For this review, take the finished solid that the model builds, in its own axes (mm). A direction names the side the tool comes from. Coordinates: 2 decimals unless noted, no trailing zeros. Loops run counter-clockwise (first coordinate to the right, second up) from the corner with the lowest first, then second, coordinate; pieces in that order, holes last. Notation, with made-up numbers: (78.25, 26.25) -> (111.25, 26.25) arc R21 cw to (111.25, 62.25) -> close; hole circle Ø4 at (-25.75, -17). An arc over 180 degrees is marked (long way). Use a Markdown table: item, result.
from build123d import *

# Parameters (mm, degrees)
SKETCH1_W               = 203.2
SKETCH1_H               = 0.889
SKETCH2_W               = 101.6
SKETCH2_H               = 16.721370504
CUT_EXTRUDE1_DEPTH      = 10.525
CUT_EXTRUDE1_DEPTH_BACK = 10.525


with BuildPart() as part:
    # Sketch1 → Revolve1 (revolve)
    with BuildSketch(Plane(origin=(0, 0, 0), x_dir=(1, 0, 0), z_dir=(0, 1, 0))):
        with Locations((101.6, 9.0805)):
            Rectangle(SKETCH1_W, SKETCH1_H)
    revolve(axis=Axis((0, 0, 0), (1, 0, 0)))

    # Sketch2 → Cut-Extrude1 (cut, two sides)
    with BuildSketch(Plane.XY) as cut_extrude1_sk:
        with Locations((101.6, 8.360685252)):
            Rectangle(SKETCH2_W, SKETCH2_H)
    extrude(amount=CUT_EXTRUDE1_DEPTH, mode=Mode.SUBTRACT)
    extrude(cut_extrude1_sk.sketch, amount=-CUT_EXTRUDE1_DEPTH_BACK, mode=Mode.SUBTRACT)


solid = part.part
(1) Take a section at D-D on x = 170.5. Write out the cut boundary in (y, z) (3 decimals).
Found:
| item | result |
|---|---|
| outline | circle Ø19.05 at (0, 0); hole circle Ø17.272 at (0, 0) |
(2) For pin 1 Ø7.5 at (y, z) = (6.5, 0.5) entering from +X; pin 2 Ø3 at (x, z) = (46.5, 2) entering from +Y, all flat-tipped, find the tip position at first contact; note any pin that passes through.
Found:
| item | result |
|---|---|
| pin 1 | stops at x = 203.2 |
| pin 2 | stops at y = 9.51 |
(3) Mouldability with a two-part tool opening along X and no side actions: class faces 1 (the face through (103.02, -9.3, 2.06)), 2 (the face through (0, -8, 4)), 3 (the face through (50.8, 9, -1)) as pulls with the +X half, pulls with the -X half, needs draft (parallel to the pull), parting line crosses it, or undercut.
Found:
| item | result |
|---|---|
| face 1 | needs draft |
| face 2 | pulls with the -X half |
| face 3 | undercut |
(4) Take a section at A-A on z = 0. Write out the cut boundary in (x, y) (3 decimals), plus the area to 3 significant figures.
Found:
| item | result |
|---|---|
| outline | (0, -9.525) -> (203.2, -9.525) -> (203.2, -8.636) -> (0, -8.636) -> close; (0, 8.636) -> (50.8, 8.636) -> (50.8, 9.525) -> (0, 9.525) -> close; (152.4, 8.636) -> (203.2, 8.636) -> (203.2, 9.525) -> (152.4, 9.525) -> close |
| area | 271 mm^2 |
(5) Take a section at B-B on y = 2. Write out the cut boundary in (x, z).
Found:
| item | result |
|---|---|
| outline | (0, -9.31) -> (50.8, -9.31) -> (50.8, -8.4) -> (0, -8.4) -> close; (0, 8.4) -> (50.8, 8.4) -> (50.8, 9.31) -> (0, 9.31) -> close; (152.4, -9.31) -> (203.2, -9.31) -> (203.2, -8.4) -> (152.4, -8.4) -> close; (152.4, 8.4) -> (203.2, 8.4) -> (203.2, 9.31) -> (152.4, 9.31) -> close |
(6) Take a section at C-C on y = -6. Write out the cut boundary in (x, z).
Found:
| item | result |
|---|---|
| outline | (0, -7.4) -> (203.2, -7.4) -> (203.2, -6.21) -> (0, -6.21) -> close; (0, 6.21) -> (203.2, 6.21) -> (203.2, 7.4) -> (0, 7.4) -> close |
(7) For faces 4 (the face through (152.4, 9, 1)), 5 (the face through (103.022, -7.662, -3.985)), list the 3-axis set-ups (+Z, -Z, +X, -X, +Y, -Y) from which the entire face can be reached by the end or side of a thin tool; tool diameter is ignored.
Found:
| item | result |
|---|---|
| face 4 | +Z, -Z, +Y |
| face 5 | +X, -X |
(8) For line 1 along Z through (x, y) = (54, -0.25); line 2 along Y through (x, z) = (17.5, -0.75); line 3 along Y through (x, z) = (21, -2.25), list the stretches that pass through material, from the lowest coordinate up.
Found:
| item | result |
|---|---|
| line 1 | z = -9.52 to -8.63, 8.63 to 9.52 |
| line 2 | y = -9.5 to -8.6, 8.6 to 9.5 |
| line 3 | y = -9.26 to -8.34, 8.34 to 9.26 |
